Here's the drawing with two shaded views (mm, measured from the low corner). I have some questions. A direction names the side the tool comes from. Coordinates: 2 decimals unless noted, no trailing zeros. Order: outer loops, then holes, each group sorted by start corner. A loop starts at its lowest first (then second) coordinate and runs counter-clockwise, first axis right, second up. Notation, with made-up numbers: (66, 78) -> (81, 78) arc R15 ccw to (81, 94) -> close; hole circle Ø4 at (10.5, 33). An arc over 180 degrees is marked (long way). Answer in a Markdown table with one row per item. Add a question column.
1. Imagine slicing it at C-C on x = 19.25. Write out the boundary of the cut face in (y, z).
2. On a 3-axis mill with a long thin cutter (end or side, diameter ignored), from which of +Z, -Z, +X, -X, +Y, -Y can I reach the whole of each face in a straight line? I mean the marked faces 1, 2, 3 and 4. Say none if no direction works.
3. Imagine slicing it at B-B on z = 13.75. Write out the boundary of the cut face in (x, y).
4. Imagine slicing it at D-D on x = 9.75. Write out the boundary of the cut face in (y, z) (1 decimal).
5. Will these pins go through, and if not, where does the flat tip stop? pin 1 (6 mm diameter, centred on x = 6, z = 3, fed in from -Y); pin 2 (2 mm diameter, centred on x = 16, y = 5.5, fed in from -Z); pin 3 (2 mm diameter, centred on x = 5, y = 3, fed in from +Z); pin 4 (3.5 mm diameter, centred on y = 3, z = 6.5, fed in from -X) (1 decimal).
6. We'd pull the mould along X, two halves only. Please class the marked faces 5, 6 and 7: pulls with the +X half, pulls with the -X half, needs draft (parallel to the pull), parting line crosses it, or undercut.
7. Imagine slicing it at A-A on y = 2.25. Write out the boundary of the cut face in (x, z).
8. If I drill on line 1 along Y through (x, z) = (2.25, 2.75); line 2 along Z through (x, y) = (15.75, 6); line 3 along X through (y, z) = (6.25, 13.75) (1 decimal), over which ranges is the centre line in solid material (lowest first)? Write a range as [from, to].
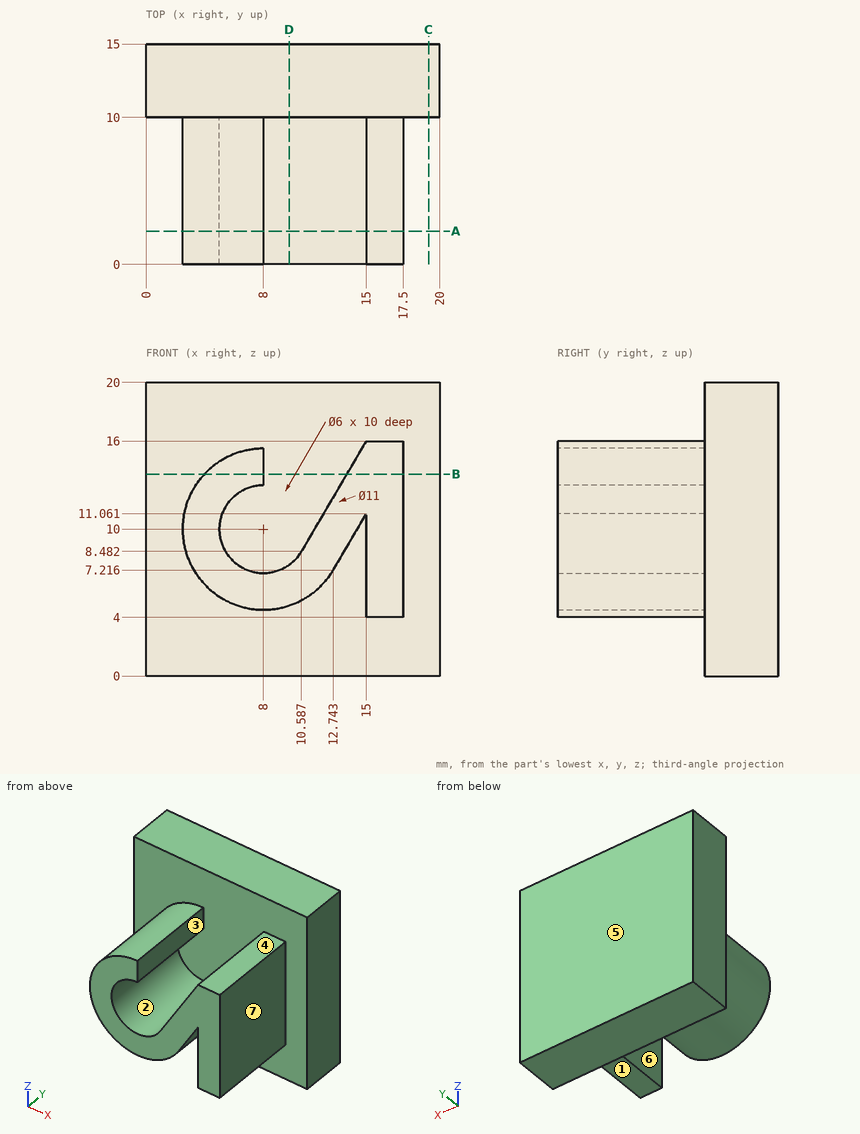
Answers follow:
| question | item | result |
|---|---|---|
| 1 | outline | (10, 0) -> (15, 0) -> (15, 20) -> (10, 20) -> close |
| 2 | face 1 | -Z, +X, -X, -Y |
| 2 | face 2 | -Y |
| 2 | face 3 | +Z, -Y |
| 2 | face 4 | +Z, +X, -X, -Y |
| 3 | outline | (0, 10) -> (3.98, 10) -> (3.98, 0) -> (8, 0) -> (8, 10) -> (13.68, 10) -> (13.68, 0) -> (17.5, 0) -> (17.5, 10) -> (20, 10) -> (20, 15) -> (0, 15) -> close |
| 4 | outline | (0, 4.8) -> (10, 4.8) -> (10, 0) -> (15, 0) -> (15, 20) -> (10, 20) -> (10, 7.6) -> (0, 7.6) -> close |
| 5 | pin 1 | stops at y = 0 |
| 5 | pin 2 | stops at z = 4 |
| 5 | pin 3 | stops at z = 15.12 |
| 5 | pin 4 | stops at x = 2.8 |
| 6 | face 5 | needs draft |
| 6 | face 6 | undercut |
| 6 | face 7 | pulls with the +X half |
| 7 | outline | (8, 13) -> (8, 15.5) arc R5.5 ccw (long way) to (12.74, 7.22) -> (15, 11.06) -> (15, 4) -> (17.5, 4) -> (17.5, 16) -> (15, 16) -> (10.59, 8.48) arc R3 cw (long way) to start |
| 8 | line 1 | y = [10, 15] |
| 8 | line 2 | z = [4, 16] |
| 8 | line 3 | x = [4, 8], [13.7, 17.5] |
